Part model, mm, in its own coordinate system. Face numbers are marked on the shaded views. A direction names the side the tool comes from. Round coordinates to 2 decimals unless told otherwise and drop trailing zeros. Write each loop counter-clockwise with the first axis right and the second up, starting at its lowest first coordinate (ties: lowest second). Pieces come first, ordered by that corner, then holes. Notation, with made-up numbers: (19.25, -20.75) -> (62.25, -20.75) arc R15 cw to (62.25, -1.75) -> close; hole circle Ø7 at (16.5, -28). An arc over 180 degrees is marked (long way). Return JSON: item names as keys, results as strings. Group by question number.
(1) Saw through at D-D (y = 7.75). List the corners of the cut face in (x, z).
(2) Tool access for the marked faces 4 and 5: list every direction of +Z, -Z, +X, -X, +Y, -Y with a clear straight run to the whole face (end or side of a thin tool).
(3) Saw through at C-C (z = 3). List the corners of the cut face in (x, y).
(4) Drill centre lines: L1, parallel to Z at x = 0, y = 11; L2, parallel to Y at x = 0.75, z = -7. Where is each one in solid material? Low to high. Write a range as from..to.
(5) Saw through at A-A (z = 0). List the corners of the cut face in (x, y).
(6) Saw through at B-B (x = 0). List the corners of the cut face in (y, z), plus the area to 3 significant figures.
(7) Drop flat-ended pins along their axis: pin 1 Ø4 at (x, z) = (0, 0) entering from +Y; pin 2 Ø4 at (x, y) = (-4, 6.5) entering from +Z; pin 3 Ø4 at (x, z) = (-6.5, -4.5) entering from -Y; pin 4 Ø6 at (y, z) = (8, -4.5) entering from -X. Give the stop position or say it passes through.
(8) Mould opens along Z. For the marked faces 1, 2 and 3 say: +Z half, -Z half, draft (parallel to the pull), parting line (faces both ways), or undercut.
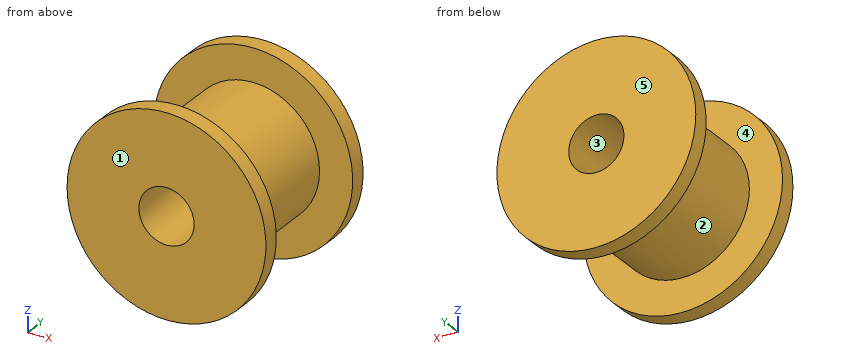
Autodesk Inventor part; units mm, degrees
ref_plane "YZ Plane" through (0, 0, 0) normal (1, 0, 0) x (0, 1, 0)
ref_plane "XZ Plane" through (0, 0, 0) normal (0, 1, 0) x (-1, 0, 0)
ref_plane "XY Plane" through (0, 0, 0) normal (0, 0, 1) x (1, 0, 0)
sketch "Sketch1" plane through (0, 0, 0) normal (0, 1, 0) x (-1, 0, 0)
  circle A0 centre (0, 0) radius 9
  dimension "d0" = 18
extrude "Extrusion1" add sketch "Sketch1" along normal blind 14
sketch "Sketch2" plane through (0, 14, 0) normal (0, 1, 0) x (1, 0, 0)
  circle A0 centre (0, 0) radius 2.5
  dimension "d3" = 5
extrude "Extrusion2" cut sketch "Sketch2" against normal through all
sketch "Sketch3" plane through (0, 0, 0) normal (1, 0, 0) x (0, 1, 0)
  line L0 (0, 0) -> (14, 0)
  line L1 (14, -9) -> (14, 9)
  line L2 (7, 0) -> (7, -9)
  line L3 (0, -9) -> (14, -9)
  line L4 (1.5, -12) -> (12.5, -12)
  line L5 (12.5, -12) -> (12.5, -6)
  line L6 (12.5, -6) -> (1.5, -6)
  line L7 (1.5, -6) -> (1.5, -12)
  line L8 (1.5, -12) -> (12.5, -6) construction
  line L9 (12.5, -12) -> (1.5, -6) construction
  dimension "d6" = 14
  dimension "d7" = 11
  dimension "d8" = 6
revolve "Revolution1" cut sketch "Sketch3" angle 360 about axis through (0, 0, 0) along (0, 1, 0) contours L6 L5 L3 L2 | L2 L3 L7 L6 | L3 L5 L4 L7
properties part number "5mm_bore_10mm_width_idlepulley"
Computed values:
{
 "1": {"outline": "circle Ø12 at (0, 0); hole circle Ø5 at (0, 0)"},
 "2": {"face 4": "none", "face 5": "+Z, -Z, +X, -X, +Y"},
 "3": {"outline": "(-8.49, 0) -> (8.49, 0) -> (8.49, 1.5) -> (5.2, 1.5) -> (5.2, 12.5) -> (8.49, 12.5) -> (8.49, 14) -> (-8.49, 14) -> (-8.49, 12.5) -> (-5.2, 12.5) -> (-5.2, 1.5) -> (-8.49, 1.5) -> close"},
 "4": {"L1": "-6..-2.5, 2.5..6", "L2": "0..1.5, 12.5..14"},
 "5": {"outline": "(-9, 0) -> (-2.5, 0) -> (-2.5, 14) -> (-9, 14) -> (-9, 12.5) -> (-6, 12.5) -> (-6, 1.5) -> (-9, 1.5) -> close; (2.5, 0) -> (9, 0) -> (9, 1.5) -> (6, 1.5) -> (6, 12.5) -> (9, 12.5) -> (9, 14) -> (2.5, 14) -> close"},
 "6": {"outline": "(0, -9) -> (1.5, -9) -> (1.5, -6) -> (12.5, -6) -> (12.5, -9) -> (14, -9) -> (14, -2.5) -> (0, -2.5) -> close; (0, 2.5) -> (14, 2.5) -> (14, 9) -> (12.5, 9) -> (12.5, 6) -> (1.5, 6) -> (1.5, 9) -> (0, 9) -> close", "area": "116 mm2"},
 "7": {"pin 1": "through", "pin 2": "z = 5.66", "pin 3": "y = 0", "pin 4": "x = -5.81"},
 "8": {"face 1": "draft", "face 2": "parting line", "face 3": "undercut"}
}
